from build123d import *

# Parameters (mm, degrees)
F0_R     = 69.85
F1_DEPTH = 2438.4
F2_R     = 50.8
F3_DEPTH = 2413
F5_DEPTH = 2336.8


with BuildPart() as f1:
    # F0 (on Top) → F1 (new body)
    with BuildSketch(Plane.XY):
        Circle(F0_R)
    extrude(amount=F1_DEPTH)

    # F2 (on face) → F3 (cut)
    with BuildSketch(Plane(origin=(0, 0, 0), x_dir=(1, 0, 0), z_dir=(0, 0, -1))):
        Circle(F2_R)
    extrude(amount=-F3_DEPTH, mode=Mode.SUBTRACT)

    # F4 (on face) → F5 (cut)
    with BuildSketch(Plane(origin=(0, 0, 0), x_dir=(1, 0, 0), z_dir=(0, 0, -1))):
        with BuildLine():
            Line((-39.655737, 31.75), (-39.655737, 57.501696))
            ThreePointArc((-39.655737, 57.501696), (-69.85, 0), (-39.655737, -57.501696))
            Line((-39.655737, -57.501696), (-39.655737, -31.75))
            Line((-39.655737, -31.75), (-39.655737, 31.75))
        make_face()
    extrude(amount=-F5_DEPTH, mode=Mode.SUBTRACT)


solid = f1.part
The listing builds one solid part. Answer for the finished solid, in the listing's coordinates (mm). A direction names the side the tool comes from. Coordinates: 2 decimals unless noted, no trailing zeros. Write each loop counter-clockwise with the first axis right and the second up, starting at its lowest first coordinate (ties: lowest second). Pieces come first, ordered by that corner, then holes. Notation, with made-up numbers: (8.5, -39.75) - (15.5, -39.75) arc R17 ccw to (15.5, -35.75) - close; hole circle Ø1 at (-34, 3). An arc over 180 degrees is marked (long way). Return JSON: item names as keys, results as strings.
1. The part is cut by section A-A on y = 0. Determine the outline of the cut face in (x, z), then the cut area to 3 significant figures.
Final values:
{"outline": "(-69.85, 2336.8) - (-50.8, 2336.8) - (-50.8, 2413) - (50.8, 2413) - (50.8, 0) - (69.85, 0) - (69.85, 2438.4) - (-69.85, 2438.4) - close", "area": "51,000 mm^2"}
2. The part is cut by section B-B on x = 0. Determine the outline of the cut face in (y, z), then the cut area to 3 significant figures.
Final values:
{"outline": "(-69.85, 0) - (-50.8, 0) - (-50.8, 2413) - (50.8, 2413) - (50.8, 0) - (69.85, 0) - (69.85, 2438.4) - (-69.85, 2438.4) - close", "area": "95,500 mm^2"}
3. Each of these flat-tipped pins is pushed along its axis until it touches: pin 1 Ø8 at (x, y) = (-0.5, 43) entering from -Z; pin 2 Ø2 at (x, z) = (28.5, 1569) entering from +Y; pin 3 Ø1 at (y, z) = (55, 1767.5) entering from +X. Where does it stop, or does it pass through?
Final values:
{"pin 1": "z = 2413", "pin 2": "y = 64.21", "pin 3": "x = 43.69"}
4. For a pull along Y with two mould halves and no side action, classify faces 1 (the face through (-1, 1, 2438.4)), 2 (the face through (64.524, -26.753, 1202.131)), 3 (the face through (48.454, -15.259, 1189.609)) as +Y half, -Y half, draft (parallel to the pull), parting line (faces both ways), or undercut.
Final values:
{"face 1": "draft", "face 2": "parting line", "face 3": "undercut"}
5. Consider line 1 along Y through (x, z) = (0, 1463); line 2 along X through (y, z) = (0, 1203); line 3 along Z through (x, y) = (-32.5, -35.5). Determine where each line is inside the solid, lowest interval first.
Final values:
{"line 1": "-69.85 to -50.8, 50.8 to 69.85", "line 2": "50.8 to 69.85", "line 3": "2413 to 2438.4"}
6. Which of the six approach directions +Z, -Z, +X, -X, +Y, -Y give full straight-line access (tool end or side, diameter ignored) to faces 4 (the face through (51, 6, 0)), 5 (the face through (-1, -1, 2413))?
Final values:
{"face 4": "-Z, +X, -X, +Y, -Y", "face 5": "-Z"}
7. The part is cut by section C-C on z = 1030. Determine the outline of the cut face in (x, y), then the cut area to 3 significant figures.
Final values:
{"outline": "(-39.66, -57.5) arc R69.85 ccw (long way) to (-39.66, 57.5) - (-39.66, 31.75) arc R50.8 cw (long way) to (-39.66, -31.75) - close", "area": "5,270 mm^2"}
